The model under review builds one solid part; all positions refer to its coordinate system, in mm. A direction names the side the tool comes from. Give positions to 0.01 mm unless a question says otherwise; leave off trailing zeros. Order: outer loops, then holes, each group sorted by start corner. A loop starts at its lowest first (then second) coordinate and runs counter-clockwise, first axis right, second up. Notation, with made-up numbers: (89.25, 34) - (117.25, 34) arc R10 cw to (117.25, 42) - close; hole circle Ø3 at (-1.5, 44.5). An arc over 180 degrees is marked (long way). Put each result on its own line as item: value.
Autodesk Inventor part; units mm, degrees
ref_plane "YZ Plane" through (0, 0, 0) normal (1, 0, 0) x (0, 1, 0)
ref_plane "XZ Plane" through (0, 0, 0) normal (0, 1, 0) x (-1, 0, 0)
ref_plane "XY Plane" through (0, 0, 0) normal (0, 0, 1) x (1, 0, 0)
ref_plane "Work Plane5" through (0, 3, 0) normal (0, 1, 0) x (1, 0, 0)
sketch "Sketch2" plane through (0, 3, 0) normal (0, 1, 0) x (1, 0, 0)
  line L0 (0, 0) -> (-19.2836, -22.9813) construction
  line L1 (5.1953, 21.7488) -> (-12.0407, 36.2115) construction
  arc A0 (-95.8881, -58.7026) -> (-19.2836, -22.9813) centre (-95.8881, 41.2974) ccw construction
  line L2 (-19.2836, -22.9813) -> (-95.8881, 41.2974) construction
  line L3 (-95.8881, 41.2974) -> (-95.8881, -58.7026) construction
  line L4 (0, 0) -> (0, -11) construction
  line L5 (6.4279, 7.6604) -> (0, 0) construction
  arc A1 (6.4279, 7.6604) -> (5.1953, 21.7488) centre (-1.2326, 14.0883) ccw construction
  arc A2 (-95.8881, -54.7026) -> (-95.8881, -62.7026) centre (-95.8881, -58.7026) ccw
  arc A3 (-95.8881, -62.7026) -> (-16.2195, -25.5525) centre (-95.8881, 41.2974) ccw
  arc A4 (-95.8881, -54.7026) -> (-22.3478, -20.4102) centre (-95.8881, 41.2974) ccw
  line L6 (-19.2836, -22.9813) -> (-22.3478, -20.4102) construction
  line L7 (-19.2836, -22.9813) -> (-16.2195, -25.5525) construction
  line L8 (10.8306, 22.2418) -> (-9.4695, 39.2757)
  arc A5 (-9.4695, 39.2757) -> (-14.6118, 33.1473) centre (-12.0407, 36.2115) ccw
  line L9 (-0.44, 21.2557) -> (-14.6118, 33.1473)
  arc A6 (2.0873, 18.0456) -> (-0.44, 21.2557) centre (-6.8679, 13.5953) ccw
  arc A7 (12.0632, 8.1535) -> (10.8306, 22.2418) centre (4.4028, 14.5813) ccw
  circle A8 centre (0, 0) radius 7 construction
  arc A9 (-1.1061, -10.9442) -> (10.5859, 2.9897) centre (0, 0) ccw
  arc A10 (-1.6433, 10.8766) -> (-10.5859, -2.9897) centre (0, 0) ccw
  line L10 (-16.2195, -25.5525) -> (-5.4391, -12.705)
  line L11 (11.5675, 7.5627) -> (12.0632, 8.1535)
  line L12 (-22.3478, -20.4102) -> (-11.5675, -7.5627)
  arc A11 (-1.1061, -10.9442) -> (-5.4391, -12.705) centre (-1.6089, -15.9189) ccw
  arc A12 (11.5675, 7.5627) -> (10.5859, 2.9897) centre (15.3977, 4.3487) ccw
  arc A13 (-11.5675, -7.5627) -> (-10.5859, -2.9897) centre (-15.3977, -4.3487) ccw
  arc A14 (-1.6433, 10.8766) -> (2.0873, 18.0456) centre (-2.3903, 15.8204) ccw
  circle A15 centre (-6.9734, -0.6101) radius 1.5 construction
  line L13 (0, 0) -> (-6.9734, -0.6101) construction
  circle A16 centre (0.6101, -6.9734) radius 1.5 construction
  circle A17 centre (6.9734, 0.6101) radius 1.5 construction
  circle A18 centre (-0.6101, 6.9734) radius 1.5 construction
  line L14 (2.9792, -2.4999) -> (-2.4999, -2.9792)
  line L15 (-2.4999, -2.9792) -> (-2.9792, 2.4999)
  line L16 (-2.9792, 2.4999) -> (2.4999, 2.9792)
  line L17 (2.4999, 2.9792) -> (2.9792, -2.4999)
  line L18 (2.9792, -2.4999) -> (-2.9792, 2.4999) construction
  line L19 (-2.4999, -2.9792) -> (2.4999, 2.9792) construction
  line L20 (-2.7395, -0.2397) -> (0, 0) construction
  point P0 (12.8558, 15.3209)
  point P1 (-3.5224, -10.4208)
  point P2 (9.6508, 5.2785)
  dimension "d53" = 14
  dimension "d24" = 30
  dimension "d27" = 32.5
  dimension "d28" = 20
  dimension "d29" = 100
  dimension "d30" = 50
  dimension "d41" = 10
  dimension "d42" = 140
  dimension "d50" = 8
  dimension "d51" = 4
  dimension "d52" = 10
  dimension "d55" = 11
  dimension "d56" = 11
  dimension "d57" = 5
  dimension "d62" = 3
  dimension "d63" = 45
  dimension "d66" = 360
  dimension "d69" = 5.5
extrude "Extrusion2" add sketch "Sketch2" along normal blind 2
chamfer "Faza1" distance 0.5 angle 45 4 edges at (2.4999, 4, -2.9792) (-2.9792, 4, -2.4999) (-2.4999, 4, 2.9792) (2.9792, 4, 2.4999)
sketch "Sketch3" plane through (0, 5, 0) normal (0, 1, 0) x (1, 0, 0)
  arc A0 (-95.8881, -54.7026) -> (-22.3478, -20.4102) centre (-95.8881, 41.2974) ccw construction
  arc A1 (-84.2223, -58.0198) -> (-17.4113, -20.6815) centre (-95.8881, 41.2974) ccw construction
  arc A2 (-95.8881, -62.7026) -> (-16.2195, -25.5525) centre (-95.8881, 41.2974) ccw construction
  line L0 (-84.2223, -58.0198) -> (-95.8881, 41.2974) construction
  line L1 (-95.8881, 41.2974) -> (-17.4113, -20.6815) construction
  line L2 (-95.8881, 41.2974) -> (0, 0) construction
  point P0 (-47.1033, -45.9954)
  dimension "d73" = 4
  dimension "d74" = 45
  dimension "d75" = 15
hole "Hole1" at (-84.2223, 5, 58.0198) at (-17.4113, 5, 20.6815) at (-47.1033, 5, 45.9954) direction (0, -1, 0) diameter 3.2 end through all
sketch "Sketch4" plane through (0, 5, 0) normal (0, 1, 0) x (1, 0, 0)
  circle A0 centre (-17.4113, -20.6815) radius 1.6
  circle A1 centre (-84.2223, -58.0198) radius 1.6
  circle A2 centre (-47.1033, -45.9954) radius 1.6
  line L0 (-2.5434, -2.4811) -> (-2.9356, 2.0018)
  line L1 (-2.4811, 2.5434) -> (-2.9356, 2.0018)
  line L2 (-2.4811, 2.5434) -> (2.0018, 2.9356)
  line L3 (2.5434, 2.4811) -> (2.0018, 2.9356)
  line L4 (2.5434, 2.4811) -> (2.9356, -2.0018)
  line L5 (2.4811, -2.5434) -> (2.9356, -2.0018)
  line L6 (2.4811, -2.5434) -> (-2.0018, -2.9356)
  line L7 (-2.5434, -2.4811) -> (-2.0018, -2.9356)
  arc A3 (-95.8881, -62.7026) -> (-16.2195, -25.5525) centre (-95.8881, 41.2974) ccw
  line L8 (-16.2195, -25.5525) -> (-5.4391, -12.705)
  arc A4 (-1.1061, -10.9442) -> (-5.4391, -12.705) centre (-1.6089, -15.9189) ccw
  arc A5 (-1.1061, -10.9442) -> (10.5859, 2.9897) centre (0, 0) ccw
  arc A6 (11.5675, 7.5627) -> (10.5859, 2.9897) centre (15.3977, 4.3487) ccw
  line L9 (11.5675, 7.5627) -> (12.0632, 8.1535)
  arc A7 (12.0632, 8.1535) -> (10.8306, 22.2418) centre (4.4028, 14.5813) ccw
  line L10 (10.8306, 22.2418) -> (-9.4695, 39.2757)
  arc A8 (-9.4695, 39.2757) -> (-14.6118, 33.1473) centre (-12.0407, 36.2115) ccw
  line L11 (-14.6118, 33.1473) -> (-0.44, 21.2557)
  arc A9 (2.0873, 18.0456) -> (-0.44, 21.2557) centre (-6.8679, 13.5953) ccw
  arc A10 (-1.6433, 10.8766) -> (2.0873, 18.0456) centre (-2.3903, 15.8204) ccw
  arc A11 (-1.6433, 10.8766) -> (-10.5859, -2.9897) centre (0, 0) ccw
  arc A12 (-11.5675, -7.5627) -> (-10.5859, -2.9897) centre (-15.3977, -4.3487) ccw
  line L12 (-11.5675, -7.5627) -> (-22.3478, -20.4102)
  arc A13 (-95.8881, -54.7026) -> (-22.3478, -20.4102) centre (-95.8881, 41.2974) ccw
  arc A14 (-95.8881, -54.7026) -> (-95.8881, -62.7026) centre (-95.8881, -58.7026) ccw
  point P0 (0, 0)
properties part number "wstepna_geometria_wersja_2"
(1) Take a section at B-B, the plane z = 0. Write out the cut boundary in (x, y), then the cut area to 3 significant figures.
The answers:
outline: (-11, 3) - (-2.76, 3) - (-2.76, 5) - (-11, 5) - close; (2.76, 3) - (11, 3) - (11, 5) - (2.76, 5) - close
area: 33.0 mm^2
(2) Take a section at A-A, the plane x = -7. Write out the cut boundary in (y, z).
The answers:
outline: (3, -37.2) - (5, -37.2) - (5, -26.76) - (3, -26.76) - close; (3, -8.49) - (5, -8.49) - (5, 14.57) - (3, 14.57) - close
(3) For faces 5 (the flat face through (-17.033, 3.986, 14.076)), 6 (the cylindrical face through (-15.161, 3.986, -38.715)), list the 3-axis set-ups (+Z, -Z, +X, -X, +Y, -Y) from which the entire face can be reached by the end or side of a thin tool; tool diameter is ignored.
The answers:
face 5: -X, +Y, -Y
face 6: +Y, -Y
(4) Take a section at D-D, the plane z = -23.5. Write out the cut boundary in (x, y).
The answers:
outline: (-3.11, 3) - (9.33, 3) - (9.33, 5) - (-3.11, 5) - close
(5) Take a section at C-C, the plane y = 4. Write out the cut boundary in (x, z) (1 decimal).
The answers:
outline: (-95.9, 54.7) arc R96 cw to (-22.3, 20.4) - (-11.6, 7.6) arc R5 cw to (-10.6, 3) arc R11 ccw to (-1.6, -10.9) arc R5 cw to (2.1, -18) arc R10 cw to (-0.4, -21.3) - (-14.6, -33.1) arc R4 ccw to (-9.5, -39.3) - (10.8, -22.2) arc R10 ccw to (12.1, -8.2) - (11.6, -7.6) arc R5 cw to (10.6, -3) arc R11 ccw to (-1.1, 10.9) arc R5 cw to (-5.4, 12.7) - (-16.2, 25.6) arc R104 ccw to (-95.9, 62.7) arc R4 ccw to start; hole circle Ø3.2 at (-84.2, 58); hole circle Ø3.2 at (-47.1, 46); hole circle Ø3.2 at (-17.4, 20.7); hole (-2.9, -2) - (-2.5, -2.5) - (2, -2.9) - (2.5, -2.5) - (2.9, 2) - (2.5, 2.5) - (-2, 2.9) - (-2.5, 2.5) - close
(6) Clearance check with flat-ended pins moving along their axes: pin 1 Ø4 at (x, z) = (-84.22, 58.02) entering from -Y; pin 2 Ø1 at (x, y) = (-12, 4.5) entering from +Z. State where each tip first meets the part, or that it passes through.
The answers:
pin 1: y = 3
pin 2: z = 21.12
(7) Wall thickness on L1, parallel to Z at x = 2, y = 3.6; L2, parallel to Z at x = -83, y = 3.35; L3, parallel to X at y = 4.85, z = -14: over which ranges is each line inside the solid? List them lowest first.
The answers:
L1: -29.65 to -18.22, -13.43 to -2.94, 2.59 to 10.82
L2: 53.83 to 56.99, 59.05 to 61.9
L3: 2.27 to 14.39
(8) The part is to be moulded in two halves that separate along X. For faces 1 (the cylindrical face through (-82.803, 3.986, 58.758)), 2 (the flat face through (-22, 3, 22)), 3 (the cylindrical face through (-9.314, 3.986, -5.852)), 4 (the cylindrical face through (-47.2, 4, 44.4)), say which applies: pulls with the +X half, pulls with the -X half, needs draft (parallel to the pull), parting line crosses it, or undercut.
The answers:
face 1: undercut
face 2: needs draft
face 3: pulls with the -X half
face 4: undercut
